Design review of the part built by this model. Coordinates are the model's own, in mm. A direction names the side the tool comes from. Give positions to 0.01 mm unless a question says otherwise; leave off trailing zeros. Loops run counter-clockwise (first coordinate to the right, second up) from the corner with the lowest first, then second, coordinate; pieces in that order, holes last. Notation, with made-up numbers: M 17,16.25 L 44,16.25 A14 ccw 44,43.25 Z; hole C -7,-8.5 d8. An arc over 180 degrees is marked long. Use a Markdown table: item, result. Add a question column.
(1) For probe 1 along Y at (x, z) = (0, 0.7); probe 2 along Z at (x, y) = (-8, -2.75); probe 3 along Z at (x, y) = (-1.25, -1.75), list the stretches that pass through material, from the lowest coordinate up.
(2) Add section D-D, the plane y = 3.25. Give the boundary of the cut face in (x, z), then the cut area to 3 significant figures.
(3) Insertion check: pin 1 Ø5 at (x, y) = (0, -9) entering from +Z; pin 2 Ø1.5 at (x, z) = (-6.5, 2) entering from -Y; pin 3 Ø1.7 at (x, y) = (1.5, -0.5) entering from +Z. Each pin has a flat end and moves straight along its axis. Give the tip position at first contact, or say it passes through.
(4) Draft analysis for pull direction X (two halves, no side actions). For faces 3 (the face through (5.9, -0.07, 0.99)), 4 (the face through (-0.59, 4.46, 3.23)), 5 (the face through (2, 0, 0)), state which applies: pulls with the +X half, pulls with the -X half, needs draft (parallel to the pull), parting line crosses it, or undercut.
(5) Add section B-B, the plane z = 0.3. Give the boundary of the cut face in (x, y).
(6) Add section A-A, the plane x = 7.5. Give the boundary of the cut face in (y, z).
(7) For faces 1 (the face through (-1, 1, 1.5)), 2 (the face through (1, -3, 4.5)), list the 3-axis set-ups (+Z, -Z, +X, -X, +Y, -Y) from which the entire face can be reached by the end or side of a thin tool; tool diameter is ignored.
(8) Add section C-C, the plane x = 3.5. Give the boundary of the cut face in (y, z).
```python
from build123d import *

# Parameters (mm, degrees)
F0_R            = 12
F1_DEPTH        = 2
F2_R            = 4.5
F3_DEPTH        = 2.5
F4_R            = 2.565
F5_DEPTH        = 3
F7_DEPTH        = 3
F7_COPIES_COUNT = 24
F8_R            = 1.25
F9_DEPTH        = 4.501
F10_R           = 1.6
F11_DEPTH       = 2


# Not quite as in the source:
# - a pattern or mirror of a feature is missing from the dataset's text; its kind, count and spacing are read off the source's solid


with BuildPart() as f1:
    # F0 (on Top) → F1 (new body)
    with BuildSketch(Plane.XY):
        Circle(F0_R)
    extrude(amount=F1_DEPTH)

    # F2 (on face) → F3 (join)
    with BuildSketch(Plane.XY.offset(2)):
        Circle(F2_R)
    extrude(amount=F3_DEPTH)

    # F4 (on face) → F5 (cut)
    with BuildSketch(Plane.XY.offset(4.5)):
        Circle(F4_R)
    extrude(amount=-F5_DEPTH, mode=Mode.SUBTRACT)

    # F6 (on face) → F7 (cut, through all)
    with BuildSketch(Plane.XY.offset(4.5)):
        with BuildLine():
            Line((0, 2.88), (-0.334799683, 2.5430560694))
            ThreePointArc((-0.334799683, 2.5430560694), (0, 2.565), (0.334799683, 2.5430560694))
            Line((0.334799683, 2.5430560694), (0, 2.88))
        make_face()
    f7 = extrude(amount=-F7_DEPTH, mode=Mode.SUBTRACT)

    # F7_copies: F7 ×24 about axis
    f7_copies_axis = Axis((0, 0, 0), (0, 0, 1))
    for i in range(1, F7_COPIES_COUNT):
        add(f7.rotate(f7_copies_axis, i * 360 / F7_COPIES_COUNT), mode=Mode.SUBTRACT)

    # F8 (on face) → F9 (cut, through all)
    with BuildSketch(Plane(origin=(0, 0, 0), x_dir=(1, 0, 0), z_dir=(0, 0, -1))):
        Circle(F8_R)
    extrude(amount=-F9_DEPTH, mode=Mode.SUBTRACT)

    # F10 (on face) → F11 (cut, through all)
    with BuildSketch(Plane(origin=(0, 0, 0), x_dir=(1, 0, 0), z_dir=(0, 0, -1))):
        with Locations((-7.5, 0)):
            Circle(F10_R)
        with Locations((7.5, 0)):
            Circle(F10_R)
    extrude(amount=-F11_DEPTH, mode=Mode.SUBTRACT)


solid = f1.part
```
Established:
| question | item | result |
|---|---|---|
| 1 | probe 1 | -12 to -1.25, 1.25 to 12 |
| 1 | probe 2 | 0 to 2 |
| 1 | probe 3 | 0 to 1.5 |
| 2 | outline | M -11.55,0 L 11.55,0 L 11.55,2 L 3.11,2 L 3.11,4.5 L -3.11,4.5 L -3.11,2 L -11.55,2 Z |
| 2 | area | 61.8 mm^2 |
| 3 | pin 1 | z = 2 |
| 3 | pin 2 | y = -10.53 |
| 3 | pin 3 | z = 1.5 |
| 4 | face 3 | undercut |
| 4 | face 4 | parting line crosses it |
| 4 | face 5 | needs draft |
| 5 | outline | C 0,0 d24; hole C -7.5,0 d3.2; hole C 0,0 d2.5; hole C 7.5,0 d3.2 |
| 6 | outline | M -9.37,0 L -1.6,0 L -1.6,2 L -9.37,2 Z; M 1.6,0 L 9.37,0 L 9.37,2 L 1.6,2 Z |
| 7 | face 1 | +Z |
| 7 | face 2 | +Z, +X, -X, +Y, -Y |
| 8 | outline | M -11.48,0 L 11.48,0 L 11.48,2 L 2.83,2 L 2.83,4.5 L -2.83,4.5 L -2.83,2 L -11.48,2 Z |
